Design review of the part built by this model. Coordinates are the model's own, in mm. Coordinates: 2 decimals unless noted, no trailing zeros. Write each loop counter-clockwise with the first axis right and the second up, starting at its lowest first coordinate (ties: lowest second). Pieces come first, ordered by that corner, then holes.
Autodesk Inventor part; units mm, degrees
ref_plane "YZ Plane" through (0, 0, 0) normal (1, 0, 0) x (0, 1, 0)
ref_plane "XZ Plane" through (0, 0, 0) normal (0, 1, 0) x (-1, 0, 0)
ref_plane "XY Plane" through (0, 0, 0) normal (0, 0, 1) x (1, 0, 0)
sketch "Sketch1" plane through (0, 0, 0) normal (0, 1, 0) x (-1, 0, 0)
  line L0 (-230, 195) -> (230, 195)
  line L1 (230, 195) -> (230, -195)
  line L2 (230, -195) -> (-230, -195)
  line L3 (-230, -195) -> (-230, 195)
  line L4 (-230, 195) -> (230, -195) construction
  line L5 (230, 195) -> (-230, -195) construction
  line L6 (210, -75) -> (210, 175)
  line L7 (210, 175) -> (-210, 175)
  line L8 (-210, 175) -> (-210, -75)
  line L9 (230, -195) -> (200, -195)
  line L10 (230, -195) -> (230, -165)
  line L11 (0, 0) -> (0, -25.7255)
  line L12 (0, 0) -> (16.1441, 0)
  circle A0 centre (200, -185) radius 2.5
  circle A1 centre (220, -165) radius 2.5
  circle A2 centre (-200, -185) radius 2.5
  circle A3 centre (-220, -165) radius 2.5
  circle A4 centre (200, 185) radius 2.5
  circle A5 centre (220, 165) radius 2.5
  circle A6 centre (-220, 165) radius 2.5
  circle A7 centre (-200, 185) radius 2.5
  line L13 (-210, 175) -> (-210, -75)
  line L14 (-210, -75) -> (210, -75)
  line L15 (206.4103, -175) -> (210, -175)
  dimension "d0" = 460
  dimension "d1" = 390
  dimension "d6" = 30
  dimension "d10" = 250
extrude "Extrusion1" add sketch "Sketch1" along normal blind 3
properties part number "TapaFrontal"
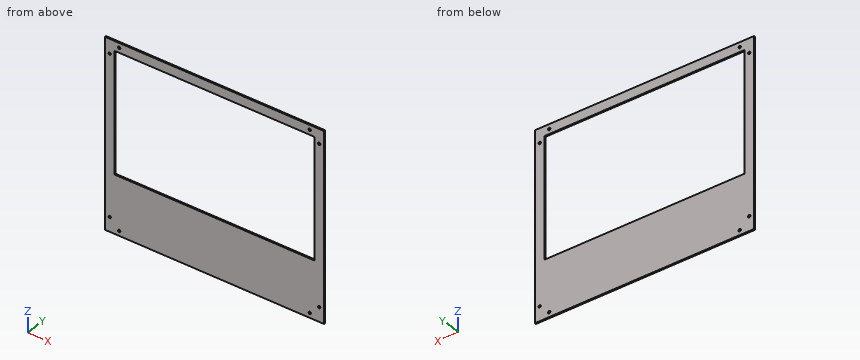
(1) Wall thickness on line 1 (Z direction, x = 200, y = 1.75); line 2 (X direction, y = 1.7, z = 185); line 3 (Z direction, x = -220, y = 1.7): over which ranges is each line inside the solid? List them lowest first.
(2) Consider section B-B (x = -154). Give the boundary of the cut face in (y, z), plus the area to 3 significant figures.
(3) Consider section A-A (z = -40.5). Give the boundary of the cut face in (x, y), plus the area to 3 significant figures.
(4) Consider section C-C (y = 1.25). State how many separate pieces and enclosed holes the cut face has, plus the area to 3 significant figures.
(5) Insertion check: pin 1 Ø4 at (x, z) = (-200, 185) entering from +Y. The pin has a flat end and moves straight along its axis. Give the tip position at first contact, or say it passes through.
Results:
1. line 1: z = -195 to -187.5, -182.5 to -75, 175 to 182.5, 187.5 to 195
1. line 2: x = -230 to -202.5, -197.5 to 197.5, 202.5 to 230
1. line 3: z = -195 to -167.5, -162.5 to 162.5, 167.5 to 195
2. outline: (0, -195) - (3, -195) - (3, -75) - (0, -75) - close; (0, 175) - (3, 175) - (3, 195) - (0, 195) - close
2. area: 420 mm2
3. outline: (-230, 0) - (-210, 0) - (-210, 3) - (-230, 3) - close; (210, 0) - (230, 0) - (230, 3) - (210, 3) - close
3. area: 120 mm2
4. separate pieces: 1
4. enclosed holes: 9
4. area: 74,200 mm2
5. pin 1: passes through
